Here's how the part is built. I have some questions about the finished solid (model axes, mm). Face numbers are marked on the shaded views. A direction names the side the tool comes from. Give positions to 0.01 mm unless a question says otherwise; leave off trailing zeros. Loops run counter-clockwise (first coordinate to the right, second up) from the corner with the lowest first, then second, coordinate; pieces in that order, holes last. Notation, with made-up numbers: (69.5, -35.75) - (116.5, -35.75) arc R5 ccw to (116.5, -31.75) - close; hole circle Ø7 at (13.25, -12.75). An arc over 180 degrees is marked (long way). Use one line per item in the form item = value.
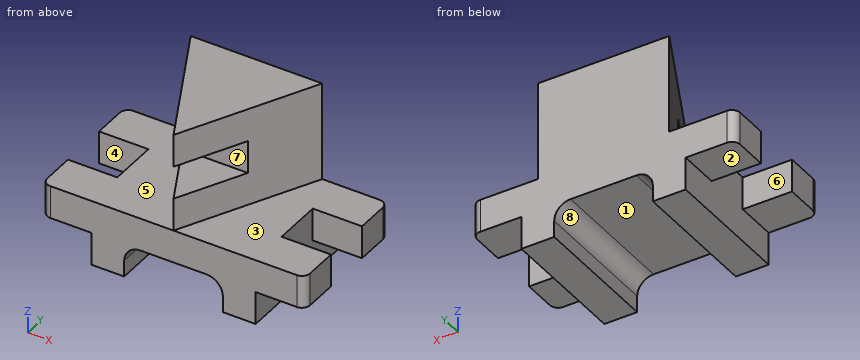
from build123d import *

# Parameters (mm, degrees)
F1_DEPTH = 101.6
F3_DEPTH = 25.4
F5_DEPTH = 76.2
F6_W     = 50.8
F6_H     = 25.4
F7_DEPTH = 165.101
F8_W     = 38.1
F8_H     = 38.1
F9_DEPTH = 50.801


with BuildPart() as f1:
    # F0 (on Front) → F1 (new body)
    with BuildSketch(Plane.XZ):
        with BuildLine():
            Line((127, 50.8), (0, 50.8))
            Line((0, 50.8), (0, 0))
            Line((0, 0), (25.4, 0))
            Line((25.4, 0), (25.4, 12.7))
            ThreePointArc((25.4, 12.7), (29.119744, 21.680256), (38.1, 25.4))
            Line((38.1, 25.4), (88.9, 25.4))
            ThreePointArc((88.9, 25.4), (97.880256, 21.680256), (101.6, 12.7))
            Line((101.6, 12.7), (101.6, 0))
            Line((101.6, 0), (127, 0))
            Line((127, 0), (127, 50.8))
        make_face()
    extrude(amount=F1_DEPTH)

    # F2 (on face) → F3 (join)
    with BuildSketch(Plane.XY.offset(50.8)):
        with BuildLine():
            Line((0, -101.6), (0, 0))
            Line((0, 0), (-31.75, 0))
            ThreePointArc((-31.75, 0), (-36.240128, -1.859872), (-38.1, -6.35))
            Line((-38.1, -6.35), (-38.1, -95.25))
            ThreePointArc((-38.1, -95.25), (-36.240128, -99.740128), (-31.75, -101.6))
            Line((-31.75, -101.6), (0, -101.6))
        make_face()
        with BuildLine():
            Line((127, 0), (127, -101.6))
            Line((127, -101.6), (158.75, -101.6))
            ThreePointArc((158.75, -101.6), (163.240128, -99.740128), (165.1, -95.25))
            Line((165.1, -95.25), (165.1, -6.35))
            ThreePointArc((165.1, -6.35), (163.240128, -1.859872), (158.75, 0))
            Line((158.75, 0), (127, 0))
        make_face()
    extrude(amount=-F3_DEPTH)

    # F4 (on face) → F5 (join)
    with BuildSketch(Plane.XY.offset(50.8)):
        Polygon((114.3, 0), (12.7, 0), (63.5, -101.6), align=None)
    extrude(amount=F5_DEPTH)

    # F6 (on Right) → F7 (cut, through all)
    with BuildSketch(Plane.YZ):
        with Locations((-76.2, 88.9)):
            Rectangle(F6_W, F6_H)
    extrude(amount=F7_DEPTH, mode=Mode.SUBTRACT)

    # F8 (on face) → F9 (cut, through all)
    with BuildSketch(Plane.XY.offset(50.8)):
        with Locations((146.05, -50.8)):
            Rectangle(F8_W, F8_H)
        with Locations((-19.05, -50.8)):
            Rectangle(F8_W, F8_H)
    extrude(amount=-F9_DEPTH, mode=Mode.SUBTRACT)


solid = f1.part
(1) If we section it at B-B (z = 8): List the corners of the cut face in (x, y) for me, plus the area to 3 significant figures.
Geometry says:
outline = (0, -101.6) - (25.4, -101.6) - (25.4, 0) - (0, 0) - close; (101.6, -101.6) - (127, -101.6) - (127, 0) - (101.6, 0) - close
area = 5,160 mm²
(2) If we section it at C-C (x = 75): List the corners of the cut face in (y, z) for me.
Geometry says:
outline = (-101.6, 25.4) - (0, 25.4) - (0, 127) - (-78.6, 127) - (-78.6, 101.6) - (-50.8, 101.6) - (-50.8, 76.2) - (-78.6, 76.2) - (-78.6, 50.8) - (-101.6, 50.8) - close
(3) Thinking about a two-plate mould opening in Y: for the marked faces 6, 7 and 8, which applies, pulls with the +Y half, pulls with the -Y half, needs draft (parallel to the pull), parting line crosses it, or undercut?
Geometry says:
face_6 = undercut
face_7 = pulls with the -Y half
face_8 = needs draft
(4) If I drill on probe 1 along Y at (x, z) = (-24, 33); probe 2 along Z at (x, y) = (114.5, -65), over which ranges is the centre line in solid material (lowest first)?
Geometry says:
probe_1 = -101.6 to -69.85, -31.75 to 0
probe_2 = 0 to 50.8
(5) If we section it at D-D (x = 131): List the corners of the cut face in (y, z) for me.
Geometry says:
outline = (-101.6, 25.4) - (-69.85, 25.4) - (-69.85, 50.8) - (-101.6, 50.8) - close; (-31.75, 25.4) - (0, 25.4) - (0, 50.8) - (-31.75, 50.8) - close
(6) For P1, Ø10, axis at y = -27, z = 8, coming from the +X side; P2, Ø14, axis at y = -72, z = 5.5, coming from the -X side; P3, Ø3, axis at y = -51, z = 81.5, coming from the -X side; P4, Ø3, axis at x = 21, z = 14.5, coming from the +Y side, each with a flat end and sliding along its axis, tell me the tip position at first contact or that it passes through.
Geometry says:
P1 = 127
P2 = 0
P3 = 37.45
P4 = 0
(7) If we section it at A-A (y = -60.5): List the corners of the cut face in (x, z) for me.
Geometry says:
outline = (0, 0) - (25.4, 0) - (25.4, 12.7) arc R12.7 cw to (38.1, 25.4) - (88.9, 25.4) arc R12.7 cw to (101.6, 12.7) - (101.6, 0) - (127, 0) - (127, 50.8) - (84.05, 50.8) - (84.05, 76.2) - (42.95, 76.2) - (42.95, 50.8) - (0, 50.8) - close; (42.95, 101.6) - (84.05, 101.6) - (84.05, 127) - (42.95, 127) - close
(8) For the marked faces 1, 2, 3, 4 and 5, which set-ups out of +Z, -Z, +X, -X, +Y, -Y let a thin tool reach every point of the face, with its end or its side?
Geometry says:
face_1 = -Z, +Y, -Y
face_2 = -Z, -X, +Y, -Y
face_3 = +Z, +X, -Y
face_4 = +Z, -Z, -X
face_5 = +Z, -X, -Y
